```python
from build123d import *

# Parameters (mm, degrees)
BASE_EXTRUDE_DEPTH = 3


with BuildPart() as part:
    # Sketch1 → Base-Extrude (new body)
    with BuildSketch(Plane.XY):
        with BuildLine():
            Line((-834.83434342, -87.678972665), (-839.364460389, -99.73670996))
            Line((-839.364460389, -99.73670996), (-842.172799168, -98.681611242))
            Line((-842.172799168, -98.681611242), (-837.642682199, -86.623873947))
            ThreePointArc((-837.642682199, -86.623873947), (-846.255704387, -95.761021528), (-852.880224121, -106.428137137))
            ThreePointArc((-852.880224121, -106.428137137), (-853.236644942, -107.398112585), (-853.386054738, -108.420641256))
            ThreePointArc((-853.386054738, -108.420641256), (-852.048634424, -112.746509925), (-848.281496833, -115.258582218))
            ThreePointArc((-848.281496833, -115.258582218), (-841.313301936, -113.662818896), (-837.190944526, -107.822581735))
            ThreePointArc((-837.190944526, -107.822581735), (-837.097500446, -107.480758655), (-836.992003912, -107.142461011))
            ThreePointArc((-836.992003912, -107.142461011), (-834.889529289, -97.524194802), (-834.83434342, -87.678972665))
        make_face()
    extrude(amount=BASE_EXTRUDE_DEPTH)


solid = part.part
```
Check sheet for the modelled part. Datum: model origin and axes. Units: mm. A direction names the side the tool comes from. Round coordinates to 2 decimals unless told otherwise and drop trailing zeros. Loops run counter-clockwise (first coordinate to the right, second up) from the corner with the lowest first, then second, coordinate; pieces in that order, holes last. Notation, with made-up numbers: (-25, -2) -> (33, -2) arc R16 cw to (33, 29) -> close; hole circle Ø4 at (75.5, 0). An arc over 180 degrees is marked (long way). Write item = value, one per line. Start each with the question number.
1) Release check for a two-part mould opening along Y. For faces 3 (the cylindrical face through (-834.905, -97.661, 1.479)), 4 (the flat face through (-844, -104, 0)), 5 (the flat face through (-840.749, -99.217, 1.479)), 6 (the flat face through (-839.94, -92.74, 1.48)) record: released by +Y, released by -Y, zero draft, split by the parting line, or undercut.
2) Sectioned sample at A-A, the plane y = -91.75. Record the cut outline in (x, z).
3) Thickness scan on probe 1 along X at (y, z) = (-95, 1); probe 2 along X at (y, z) = (-88.25, 1.4); probe 3 along X at (y, z) = (-112.75, 0.3). Record the ranges inside material, lowest first.
4) Sectioned sample at D-D, the plane x = -850.75. Record the cut outline in (y, z).
5) Sectioned sample at C-C, the plane x = -839. Record the cut outline in (y, z).
6) Set-up check for faces 1 (the flat face through (-837.068, -93.623, 1.479)), 2 (the cylindrical face through (-853.23, -107.38, 1.48)): record each of +Z, -Z, +X, -X, +Y, -Y from which the full face is reachable in a straight line by a thin tool's end or side.
7) Sectioned sample at B-B, the plane z = 1.35. Record the cut outline in (x, y), plus the area to 3 significant figures.
8) Gauge pin test, flat ends, axial feed: pin 1 Ø1.5 at (x, y) = (-844.5, -111) entering from -Z; pin 2 Ø1 at (y, z) = (-111.5, 1) entering from -X; pin 3 Ø1 at (y, z) = (-112.5, 2) entering from -X. Record the tip position at first contact, or that the pin passes through.
Results are:
q1.face_3 = split by the parting line
q1.face_4 = zero draft
q1.face_5 = undercut
q1.face_6 = undercut
q2.outline = (-842.89, 0) -> (-839.57, 0) -> (-839.57, 3) -> (-842.89, 3) -> close; (-836.36, 0) -> (-834.61, 0) -> (-834.61, 3) -> (-836.36, 3) -> close
q3.probe_1 = -845.66 to -840.79, -837.58 to -834.68
q3.probe_2 = -839.44 to -838.25, -835.05 to -834.78
q3.probe_3 = -852.05 to -840.15
q4.outline = (-114.06, 0) -> (-102.45, 0) -> (-102.45, 3) -> (-114.06, 3) -> close
q5.outline = (-111.51, 0) -> (-98.77, 0) -> (-98.77, 3) -> (-111.51, 3) -> close; (-90.24, 0) -> (-87.84, 0) -> (-87.84, 3) -> (-90.24, 3) -> close
q6.face_1 = +Z, -Z
q6.face_2 = +Z, -Z, -X, +Y
q7.outline = (-853.39, -108.42) arc R6.76 ccw to (-848.28, -115.26) arc R10 ccw to (-837.19, -107.82) arc R10 cw to (-836.99, -107.14) arc R47.06 ccw to (-834.83, -87.68) -> (-839.36, -99.74) -> (-842.17, -98.68) -> (-837.64, -86.62) arc R62.84 ccw to (-852.88, -106.43) arc R5 ccw to start
q7.area = 298 mm^2
q8.pin_1 = 0
q8.pin_2 = -852.99
q8.pin_3 = -852.53
